```python
from build123d import *

# Parameters (mm, degrees)
F0_W           = 65.5
F0_H           = 35
F0_W_2         = 17.25
F1_DEPTH       = 1.5
F2_DEPTH       = 17.5
F3_DEPTH       = 7.3
F4_R           = 4.4
F4_R_2         = 2.625
F5_DEPTH       = 55
F6_DEPTH       = 55.001
F6_DEPTH_BACK  = 55.001
F7_R           = 8.75
F9_D           = 5.6134
F9_CSINK_D     = 10.4394
F9_CSINK_ANGLE = 82


with BuildPart() as f1:
    # F0 (on Top) → F1 (new body)
    with BuildSketch(Plane.XY):
        Rectangle(F0_W, F0_H)
        with Locations((-41.375, 0)):
            Rectangle(F0_W_2, F0_H)
        with Locations((41.375, 0)):
            Rectangle(F0_W_2, F0_H)
    extrude(amount=F1_DEPTH)

    # F0 (on Top) → F2 (join)
    with BuildSketch(Plane.XY):
        with Locations((-41.375, 0)):
            Rectangle(F0_W_2, F0_H)
        with Locations((41.375, 0)):
            Rectangle(F0_W_2, F0_H)
    extrude(amount=-F2_DEPTH)

    # F0 (on Top) → F3 (join)
    with BuildSketch(Plane.XY):
        Rectangle(F0_W, F0_H)
    extrude(amount=-F3_DEPTH)

    # F4 (on Right) → F5 (join, symmetric)
    with BuildSketch(Plane.YZ):
        with Locations((0, -2.9)):
            Circle(F4_R)
        with Locations((0, -2.9)):
            Circle(F4_R_2, mode=Mode.SUBTRACT)
    extrude(amount=F5_DEPTH, both=True)

    # F4 (on Right) → F6 (cut, two sides)
    with BuildSketch(Plane.YZ) as f6_sk:
        with Locations((0, -2.9)):
            Circle(F4_R_2)
    extrude(amount=-F6_DEPTH, mode=Mode.SUBTRACT)
    extrude(f6_sk.sketch, amount=F6_DEPTH_BACK, mode=Mode.SUBTRACT)

    # F7
    f7_edges = [f1.edges().sort_by_distance(p)[0] for p in [
        (41.375, -17.5, -17.5),
        (41.375, 17.5, -17.5),
        (-41.375, -17.5, -17.5),
        (-41.375, 17.5, -17.5),
    ]]
    fillet(f7_edges, radius=F7_R)

    # F9 (through all)
    with Locations(Plane.XY.offset(1.5)):
        with Locations((-22.75, 7.5), (-22.75, -7.5), (22.75, -7.5), (22.75, 7.5)):
            CounterSinkHole(F9_D / 2, F9_CSINK_D / 2, counter_sink_angle=F9_CSINK_ANGLE)


solid = f1.part
```
Geometry check sheet. Reference: the model listing, model coordinates, mm. A direction names the side the tool comes from. Round coordinates to 2 decimals unless told otherwise and drop trailing zeros. Loops run counter-clockwise (first coordinate to the right, second up) from the corner with the lowest first, then second, coordinate; pieces in that order, holes last. Notation, with made-up numbers: (-38, 73) - (-10, 73) arc R10 ccw to (-10, 79) - close; hole circle Ø4 at (7.25, 59). An arc over 180 degrees is marked (long way). Write each question's results on one line, items separated by ' | '. Start each with the question number.
Q1. Access from +Z, -Z, +X, -X, +Y, -Y to the whole of each face (thin tool, end or side, straight path). Record for faces 1 (the flat face through (-32.75, 0, -12)), 2 (the cylindrical face through (-52.465, 2.03, -6.804)), 3 (the flat face through (-55, 2, -5)).
Q2. Gauge pin test, flat ends, axial feed: P1, Ø8, axis at y = -4, z = -11, coming from the +X side; P2, Ø10, axis at x = -7.5, y = -2, coming from the -Z side; P3, Ø10, axis at x = -22, z = -9.5, coming from the -Y side; P4, Ø3, axis at y = 3, z = -12, coming from the -X side. Record the tip position at first contact, or that the pin passes through.
Q3. Cross-section at A-A on x = -22.75. Enter the section's corners in (y, z) (3 decimals).
Q4. Cross-section at B-B on z = -2.9. Enter the section's corners in (x, y) (3 decimals), and give its area (3 significant figures).
Q5. Cross-section at C-C on x = -42.5. Enter the section's corners in (y, z) (3 decimals), and give its area (3 significant figures).
Q6. Release check for a two-part mould opening along Z. For faces 4 (the cylindrical face through (41.496, -14.869, -15.005)), 5 (the flat face through (32.75, 0, -12)), 6 (the cylindrical face through (-0.77, -0.569, -5.463)), 7 (the cylindrical face through (52.535, 2.03, -6.804)) record: +Z half, -Z half, draft (parallel to the pull), parting line (faces both ways), or undercut.
Q7. Cross-section at D-D on y = 7.5. Enter the section's corners in (x, z), and give its area (3 significant figures).
Q8. Thickness scan on line 1 (X direction, y = 7.5, z = -3); line 2 (Y direction, x = 22.75, z = -2.75); line 3 (X direction, y = -6, z = -13). Record the ranges inside material, lowest first. Write a range as [from, to].
Answers below:
1) face 1: -Z, +Y, -Y | face 2: -X | face 3: +Z, -Z, -X, +Y, -Y
2) P1: stops at x = 50 | P2: stops at z = -7.3 | P3: stops at y = -17.5 | P4: stops at x = -50
3) outline: (-17.5, -7.3) - (-10.307, -7.3) - (-10.307, -1.276) - (-12.72, 1.5) - (-17.5, 1.5) - close; (-4.693, -7.3) - (4.693, -7.3) - (4.693, -1.276) - (2.28, 1.5) - (-2.28, 1.5) - (-4.693, -1.276) - close; (10.307, -7.3) - (17.5, -7.3) - (17.5, 1.5) - (12.72, 1.5) - (10.307, -1.276) - close; hole circle Ø5.25 at (0, -2.9)
4) outline: (-55, -4.4) - (-50, -4.4) - (-50, -17.5) - (50, -17.5) - (50, -4.4) - (55, -4.4) - (55, -2.625) - (-55, -2.625) - close; (-55, 2.625) - (55, 2.625) - (55, 4.4) - (50, 4.4) - (50, 17.5) - (-50, 17.5) - (-50, 4.4) - (-55, 4.4) - close; hole circle Ø5.613 at (-22.75, -7.5); hole circle Ø5.613 at (-22.75, 7.5); hole circle Ø5.613 at (22.75, -7.5); hole circle Ø5.613 at (22.75, 7.5) | area: 2,910 mm²
5) outline: (-17.5, -8.75) arc R8.75 ccw to (-8.75, -17.5) - (8.75, -17.5) arc R8.75 ccw to (17.5, -8.75) - (17.5, 1.5) - (-17.5, 1.5) - close; hole circle Ø5.25 at (0, -2.9) | area: 610 mm²
6) face 4: -Z half | face 5: draft | face 6: undercut | face 7: parting line
7) outline: (-50, -17.5) - (-32.75, -17.5) - (-32.75, -7.3) - (-25.56, -7.3) - (-25.56, -1.28) - (-27.97, 1.5) - (-50, 1.5) - close; (-19.94, -7.3) - (19.94, -7.3) - (19.94, -1.28) - (17.53, 1.5) - (-17.53, 1.5) - (-19.94, -1.28) - close; (25.56, -7.3) - (32.75, -7.3) - (32.75, -17.5) - (50, -17.5) - (50, 1.5) - (27.97, 1.5) - (25.56, -1.28) - close | area: 1,120 mm²
8) line 1: x = [-50, -25.56], [-19.94, 19.94], [25.56, 50] | line 2: y = [-17.5, -10.31], [-4.69, -2.62], [2.62, 4.69], [10.31, 17.5] | line 3: x = [-50, -32.75], [32.75, 50]
